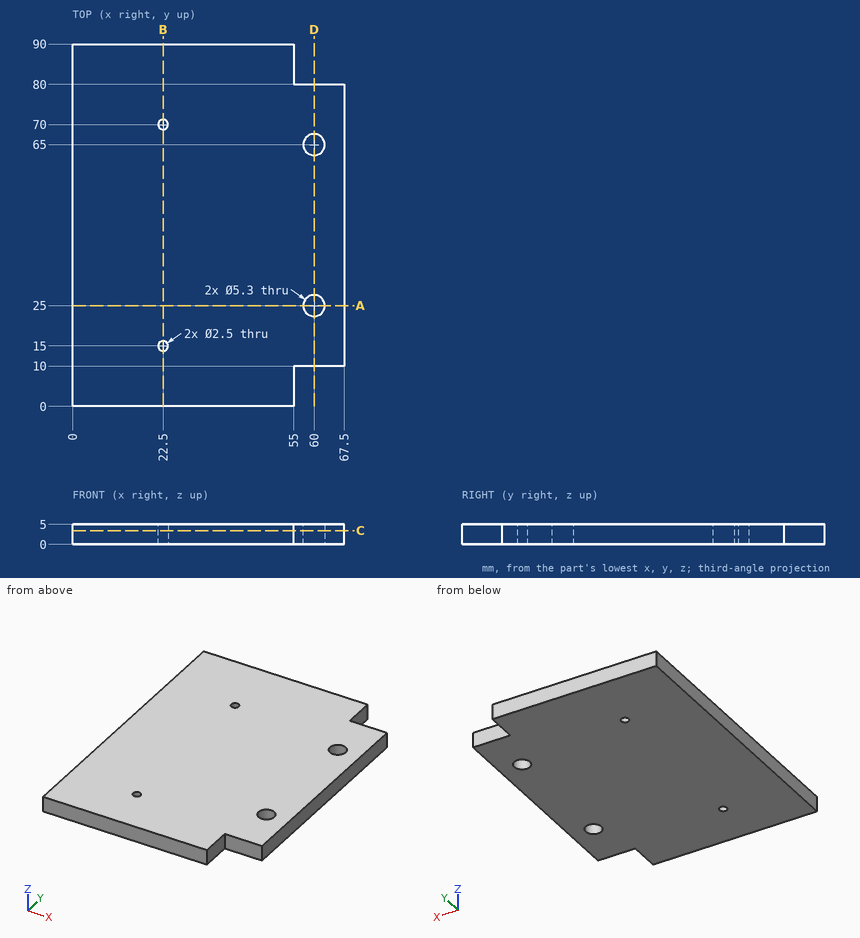
Design review of the part shown in the three views and the two pictorial views. Dimensions are in mm from the part's minimum x, y and z. Give positions to 0.01 mm unless a question says otherwise; leave off trailing zeros. Write each loop counter-clockwise with the first axis right and the second up, starting at its lowest first coordinate (ties: lowest second). Pieces come first, ordered by that corner, then holes. Notation, with made-up numbers: (80, 3.25) - (120, 3.25) arc R37 cw to (120, 39.25) - close; hole circle Ø8 at (7.25, -13.5). An arc over 180 degrees is marked (long way). Return JSON: item names as keys, results as strings. Group by question number.
(1) Insertion check: pin 1 (5 mm diameter, centred on x = 60, y = 65, fed in from +Z); pin 2 (2.5 mm diameter, centred on y = 86.5, z = 3.5, fed in from +X). Each pin has a flat end and moves straight along its axis. Give the tip position at first contact, or say it passes through.
(2) We need section D-D, the plane x = 60. Give the boundary of the cut face in (y, z).
(3) We need section C-C, the plane z = 3.4. Give the boundary of the cut face in (x, y).
(4) We need section A-A, the plane y = 25. Give the boundary of the cut face in (x, z).
(5) We need section B-B, the plane x = 22.5. Give the boundary of the cut face in (y, z), then the cut area to 3 significant figures.
(6) To check wall thickness, follow probe 1 along Y at (x, z) = (60, 3.7); probe 2 along Y at (x, z) = (22.5, 2.7); probe 3 along X at (y, z) = (84, 4.15). State the ranges of each line that lie inside material, in increasing order.
Reported:
{
 "1": {"pin 1": "passes through", "pin 2": "stops at x = 55"},
 "2": {"outline": "(10, 0) - (22.35, 0) - (22.35, 5) - (10, 5) - close; (27.65, 0) - (62.35, 0) - (62.35, 5) - (27.65, 5) - close; (67.65, 0) - (80, 0) - (80, 5) - (67.65, 5) - close"},
 "3": {"outline": "(0, 0) - (55, 0) - (55, 10) - (67.5, 10) - (67.5, 80) - (55, 80) - (55, 90) - (0, 90) - close; hole circle Ø2.5 at (22.5, 15); hole circle Ø2.5 at (22.5, 70); hole circle Ø5.3 at (60, 25); hole circle Ø5.3 at (60, 65)"},
 "4": {"outline": "(0, 0) - (57.35, 0) - (57.35, 5) - (0, 5) - close; (62.65, 0) - (67.5, 0) - (67.5, 5) - (62.65, 5) - close"},
 "5": {"outline": "(0, 0) - (13.75, 0) - (13.75, 5) - (0, 5) - close; (16.25, 0) - (68.75, 0) - (68.75, 5) - (16.25, 5) - close; (71.25, 0) - (90, 0) - (90, 5) - (71.25, 5) - close", "area": "425 mm2"},
 "6": {"probe 1": "y = 10 to 22.35, 27.65 to 62.35, 67.65 to 80", "probe 2": "y = 0 to 13.75, 16.25 to 68.75, 71.25 to 90", "probe 3": "x = 0 to 55"}
}
